Part model, mm, in its own coordinate system. A direction names the side the tool comes from. Give positions to 0.01 mm unless a question says otherwise; leave off trailing zeros. Write each loop counter-clockwise with the first axis right and the second up, starting at its lowest first coordinate (ties: lowest second). Pieces come first, ordered by that corner, then holes. Notation, with made-up numbers: M -29,1 L -22,1 A16 cw -22,22 Z; hole C 24.25,48 d5. An arc over 180 degrees is marked long. Use a Markdown table: item, result.
```python
from build123d import *

# Parameters (mm, degrees)
F0_W      = 74.2475399747
F0_H      = 85.0587636232
F1_DEPTH  = 38
F2_W      = 27.2778645158
F2_H      = 48.6257560551
F2_W_2    = 26.5662674792
F2_H_2    = 48.8629546016
F3_DEPTH  = 5.1
F4_R      = 5
F5_R      = 7.356985616
F5_R_2    = 9.8858115492
F5_R_3    = 4.3495434343
F6_DEPTH  = 3.7
F7_SIZE   = 2
F8_R      = 14.4594029366
F9_DEPTH  = 7.8
F10_R     = 19.4422944141
F11_DEPTH = 16.9
F12_W     = 43.763179332
F12_H     = 9.2507535592
F13_DEPTH = 9.1
F14_W     = 82.5197082013
F14_H     = 37.9795394838
F15_DEPTH = 59.4
F17_DEPTH = 6
F18_R     = 10.1503328775
F19_DEPTH = 2.4
F21_DEPTH = 0.8


with BuildPart() as f1:
    # F0 (on Front) → F1 (new body)
    with BuildSketch(Plane.XZ):
        with Locations((-24.6077510528, -4.1337423027)):
            Rectangle(F0_W, F0_H)
    extrude(amount=F1_DEPTH)

    # F2 (on face) → F3 (join)
    with BuildSketch(Plane.XZ.offset(38)):
        with Locations((-42.4585863948, 5.2183736116)):
            Rectangle(F2_W, F2_H)
        with Locations((-6.2857677694, 5.0997743383)):
            Rectangle(F2_W_2, F2_H_2)
    extrude(amount=F3_DEPTH)

    # F4
    f4_edges = [f1.edges().sort_by_distance(p)[0] for p in [
        (-42.458586, -43.1, 29.531252),
        (-6.285768, -43.1, 29.531252),
        (-6.285768, -43.1, -19.331703),
        (-42.458586, -43.1, -19.094504),
        (-19.568902, -43.1, 5.099774),
        (-28.819654, -43.1, 5.218374),
        (-56.097519, -43.1, 5.218374),
        (6.997366, -43.1, 5.099774),
    ]]
    fillet(f4_edges, radius=F4_R)

    # F5 (on face) → F6 (join)
    with BuildSketch(Plane.XZ.offset(38)):
        with Locations((-43.0515818298, -33.8008292019)):
            Circle(F5_R)
        with Locations((-20.9920946509, -34.9868237972)):
            Circle(F5_R_2)
        with Locations((0, -34.5124267042)):
            Circle(F5_R_3)
    extrude(amount=F6_DEPTH)

    # F7
    f7_edges = [f1.edges().sort_by_distance(p)[0] for p in [
        (-50.408567, -41.7, -33.800829),
        (-30.877906, -41.7, -34.986824),
        (-4.349543, -41.7, -34.512427),
    ]]
    chamfer(f7_edges, length=F7_SIZE)

    # F8 (on face) → F9 (join)
    with BuildSketch(Plane.YZ.offset(12.5160189345)):
        with Locations((-18.8573058695, 18.3829069138)):
            Circle(F8_R)
    extrude(amount=F9_DEPTH)

    # F10 (on face) → F11 (join)
    with BuildSketch(Plane.YZ.offset(20.3160189345)):
        with Locations((-18.8573058695, 18.3829069138)):
            Circle(F10_R)
    extrude(amount=F11_DEPTH)

    # F12 (on face) → F13 (join)
    with BuildSketch(Plane.XY.offset(38.395639509)):
        with Locations((-21.881589666, -19.687501248)):
            Rectangle(F12_W, F12_H)
    extrude(amount=F13_DEPTH)

    # F14 (on face) → F15 (join)
    with BuildSketch(Plane.XY.offset(47.495639509)):
        with Locations((-23.5268557444, -18.9897697419)):
            Rectangle(F14_W, F14_H)
    extrude(amount=F15_DEPTH)

    # F16 (on face) → F17 (cut)
    with BuildSketch(Plane.XZ.offset(37.9795394838)):
        with BuildLine():
            add(Edge.make_bspline(
                [(-26.0310750455, 66.1403313279), (-19.5197759633, 72.7342236821), (3.3929896724, 82.8686218481), (4.6264940271, 58.9542461456), (-33.4389955915, 50.822229714), (-29.9990735288, 62.122000342), (-26.0310750455, 66.1403313279)],
                knots=[0, 0, 0, 0, 0.3027684682, 0.5046913629, 0.8154922992, 1, 1, 1, 1], degree=3))
        make_face()
    extrude(amount=-F17_DEPTH, mode=Mode.SUBTRACT)

    # F18 (on face) → F19 (join)
    with BuildSketch(Plane.XZ.offset(37.9795394838)):
        with Locations((-49.7975498438, 91.5002599359)):
            Circle(F18_R)
    extrude(amount=F19_DEPTH)

    # F20 (on face) → F21 (cut)
    with BuildSketch(Plane.XZ.offset(40.3795394838)):
        Polygon((-50.9105199745, 88.8133123517), (-48.684579713, 88.8133123517), (-47.1106022596, 90.3872898051), (-47.1106022596, 92.6132300666), (-48.684579713, 94.18720752), (-50.9105199745, 94.18720752), (-52.4844974279, 92.6132300666), (-52.4844974279, 90.3872898051), align=None)
    extrude(amount=-F21_DEPTH, mode=Mode.SUBTRACT)


solid = f1.part
```
1. Drop flat-ended pins along their axis: P1, Ø6, axis at y = -34.5, z = 11.5, coming from the -X side; P2, Ø16, axis at x = -48, z = 92, coming from the -Y side; P3, Ø7.5, axis at x = -21, z = 41, coming from the +Y side. Give the stop position or say it passes through.
Findings below:
| item | result |
|---|---|
| P1 | x = -61.73 |
| P2 | y = -40.38 |
| P3 | y = 0 |
2. Drill centre lines: L1, parallel to Z at x = -34, y = -6; L2, parallel to Y at x = -9, z = 80.5; L3, parallel to X at y = -16, z = -19. Where is each one in solid material? Low to high.
Findings below:
| item | result |
|---|---|
| L1 | -46.66 to 38.4, 47.5 to 106.9 |
| L2 | -37.98 to 0 |
| L3 | -61.73 to 12.52 |
3. Two-plate mould, pull along X, no slides. Class faces 1 (the flat face through (-24, -37.98, 77)), 2 (the flat face through (-64.787, -19, 77)), 3 (the cylindrical face through (4.018, -38.838, -36.178)), 4 (the cylindrical face through (-44.34, -39.16, 100.06)): released by +X, released by -X, zero draft, split by the parting line, or undercut.
Findings below:
| item | result |
|---|---|
| face 1 | zero draft |
| face 2 | released by -X |
| face 3 | undercut |
| face 4 | split by the parting line |
4. Tool access for faces 5 (the cylindrical face through (-54.67, -41.6, 5.56)), 6 (the cylindrical face through (28.65, -38.28, 19.24)), 7 (the cylindrical face through (-44.009, -38.838, -26.506)), 8 (the flat face through (-21, -41.7, -35)), 9 (the cylindrical face through (-18.14, -41.6, 5.44)): list every direction of +Z, -Z, +X, -X, +Y, -Y with a clear straight run to the whole face (end or side of a thin tool).
Findings below:
| item | result |
|---|---|
| face 5 | -Z, -X, -Y |
| face 6 | +X |
| face 7 | -Y |
| face 8 | -Z, +X, -X, -Y |
| face 9 | +Z, -Y |
5. Cut at A-A, the plane z = 83. Give the cut face in (x, y).
Findings below:
| item | result |
|---|---|
| outline | M -64.79,-37.98 L -55.35,-37.98 L -55.35,-40.38 L -44.25,-40.38 L -44.25,-37.98 L 17.73,-37.98 L 17.73,0 L -64.79,0 Z |
6. Cut at B-B, the plane y = -18. Give the cut face in (x, z).
Findings below:
| item | result |
|---|---|
| outline | M -64.79,47.5 L -43.76,47.5 L -43.76,38.4 L -61.73,38.4 L -61.73,-46.66 L 12.52,-46.66 L 12.52,3.95 L 20.32,3.95 L 20.32,-1.04 L 37.22,-1.04 L 37.22,37.81 L 20.32,37.81 L 20.32,32.82 L 12.52,32.82 L 12.52,38.4 L 0,38.4 L 0,47.5 L 17.73,47.5 L 17.73,106.9 L -64.79,106.9 Z |
